```python
from build123d import *

# Parameters (mm, degrees)
SZKIC1_W                       = 46
SZKIC1_H                       = 76
SZKIC1_R                       = 14
DODANIE_WYCI_GNI_CIE1_DEPTH    = 35
SFAZOWANIE1_SIZE               = 1
OTW_R_GWINTOWANY_M6X1_01_D     = 5
OTW_R_GWINTOWANY_M6X1_01_DEPTH = 17
OTW_R_GWINTOWANY_M6X1_01_TIP   = 1.502151548
OTW_R_GWINTOWANY_M6X1_03_D     = 5
OTW_R_GWINTOWANY_M6X1_03_DEPTH = 17
OTW_R_GWINTOWANY_M6X1_03_TIP   = 1.502151548
SFAZOWANIE2_SIZE               = 10
WYTNIJ_WYCI_GNI_CIE1_DEPTH     = 96.482982777


with BuildPart() as part:
    # Szkic1 → Dodanie-wyciągnięcie1 (new body)
    with BuildSketch(Plane.XY):
        with Locations((23, 38)):
            Rectangle(SZKIC1_W, SZKIC1_H)
        with Locations((20.5, 38)):
            Circle(SZKIC1_R, mode=Mode.SUBTRACT)
    extrude(amount=DODANIE_WYCI_GNI_CIE1_DEPTH)

    # Sfazowanie1
    sfazowanie1_edges = [part.edges().sort_by_distance(p)[0] for p in [
        (6.5, 38, 0),
        (6.5, 38, 35),
    ]]
    chamfer(sfazowanie1_edges, length=SFAZOWANIE1_SIZE)

    # Otwór gwintowany M6x1.01
    with Locations(Plane.XY.offset(35)):
        with Locations((20.5, 57), (7.064971157, 51.435028843), (7.064971157, 24.564971157), (20.5, 19)):
            Hole(OTW_R_GWINTOWANY_M6X1_01_D / 2, depth=OTW_R_GWINTOWANY_M6X1_01_DEPTH)
            with Locations((0, 0, -(OTW_R_GWINTOWANY_M6X1_01_DEPTH + OTW_R_GWINTOWANY_M6X1_01_TIP / 2))):  # 118° drill point
                Cone(0, OTW_R_GWINTOWANY_M6X1_01_D / 2, OTW_R_GWINTOWANY_M6X1_01_TIP, mode=Mode.SUBTRACT)

    # Otwór gwintowany M6x1.03
    with Locations(Plane(origin=(46, 0, 0), x_dir=(0, 0, -1), z_dir=(1, 0, 0))):
        with Locations((-29, 70), (-6, 70), (-6, 6), (-29, 6)):
            Hole(OTW_R_GWINTOWANY_M6X1_03_D / 2, depth=OTW_R_GWINTOWANY_M6X1_03_DEPTH)
            with Locations((0, 0, -(OTW_R_GWINTOWANY_M6X1_03_DEPTH + OTW_R_GWINTOWANY_M6X1_03_TIP / 2))):  # 118° drill point
                Cone(0, OTW_R_GWINTOWANY_M6X1_03_D / 2, OTW_R_GWINTOWANY_M6X1_03_TIP, mode=Mode.SUBTRACT)

    # Sfazowanie2
    sfazowanie2_edges = [part.edges().sort_by_distance(p)[0] for p in [
        (0, 76, 17.5),
        (0, 0, 17.5),
    ]]
    chamfer(sfazowanie2_edges, length=SFAZOWANIE2_SIZE)

    # Szkic10 → Wytnij-wyciągnięcie1 (cut, through all)
    with BuildSketch(Plane(origin=(0, 0, 0), x_dir=(-1, 0, 0), z_dir=(0, 0, -1))):
        Polygon((-46, 13), (-46, 63), (-34, 63), (-34, 53), (-42, 53), (-42, 23), (-34, 23), (-34, 13), align=None)
    extrude(amount=-WYTNIJ_WYCI_GNI_CIE1_DEPTH, mode=Mode.SUBTRACT)


solid = part.part
```
Design review of the part built by this model. Coordinates are the model's own, in mm. A direction names the side the tool comes from. Coordinates: 2 decimals unless noted, no trailing zeros. Loops run counter-clockwise (first coordinate to the right, second up) from the corner with the lowest first, then second, coordinate; pieces in that order, holes last.
Q1. We need section C-C on x = 31.5. State how many separate pieces and enclosed holes the cut face has, and give its area (3 significant figures).
Reported:
separate pieces: 2
enclosed holes: 4
area: 1,970 mm2
Q2. To check wall thickness, follow line 1 (Z direction, x = 33, y = 70); line 2 (Y direction, x = 36, z = 6); line 3 (Y direction, x = 38, z = 18). State the ranges of each line that lie inside material, in increasing order.
Reported:
line 1: z = 0 to 3.5, 8.5 to 26.5, 31.5 to 35
line 2: y = 0 to 3.5, 8.5 to 13, 23 to 53, 63 to 67.5, 72.5 to 76
line 3: y = 0 to 13, 23 to 53, 63 to 76
Q3. Tool access review of faces 4 (the face through (28, 0, 17)), 5 (the face through (37.38, 67.56, 28.46)), 6 (the face through (5.91, 22.35, 26.38)), 7 (the face through (40, 63, 17)): name each direction out of +Z, -Z, +X, -X, +Y, -Y from which nothing blocks a thin tool from reaching the whole face with its end or side.
Reported:
face 4: +Z, -Z, +X, -X, -Y
face 5: +X
face 6: +Z
face 7: +Z, -Z, +X
Q4. For pin 1 (8 mm diameter, centred on y = 34.5, z = 10.5, fed in from +X); pin 2 (12 mm diameter, centred on x = 21.5, y = 45, fed in from -Z) (1 decimal); pin 3 (4 mm diameter, centred on x = 20.5, y = 19, fed in from +Z); pin 4 (4.5 mm diameter, centred on y = 6, z = 29, fed in from -X), all flat-tipped, find the tip position at first contact; note any pin that passes through.
Reported:
pin 1: stops at x = 42
pin 2: passes through
pin 3: stops at z = 17.7
pin 4: stops at x = 1.75
Q5. We need section A-A on z = 10. State the section outline as (x, y) points, and give its area (3 significant figures).
Reported:
outline: (0, 10) - (10, 0) - (46, 0) - (46, 13) - (34, 13) - (34, 23) - (42, 23) - (42, 53) - (34, 53) - (34, 63) - (46, 63) - (46, 76) - (10, 76) - (0, 66) - close; hole circle Ø28 at (20.5, 38)
area: 2,420 mm2
Q6. We need section D-D on y = 61. State the section outline as (x, z) points, and give its area (3 significant figures).
Reported:
outline: (0, 0) - (34, 0) - (34, 35) - (0, 35) - close
area: 1,190 mm2
Q7. The part is to be moulded in two halves that separate along Z. For faces 1 (the face through (20.44, 57.43, 16.76)), 2 (the face through (27.759, 69.736, 6.345)), 3 (the face through (22, 21, 26)), say which applies: +Z half, -Z half, draft (parallel to the pull), parting line (faces both ways), or undercut.
Reported:
face 1: +Z half
face 2: undercut
face 3: draft
Q8. We need section B-B on y = 38. State the section outline as (x, z) points.
Reported:
outline: (0, 0) - (5.5, 0) - (6.5, 1) - (6.5, 34) - (5.5, 35) - (0, 35) - close; (34.5, 1) - (35.5, 0) - (42, 0) - (42, 35) - (35.5, 35) - (34.5, 34) - close
